```python
from build123d import *

# Parameters (mm, degrees)
F3_DEPTH = 67


with BuildPart() as f1:
    # F0 (on Right) → F1 (revolve)
    with BuildSketch(Plane.YZ):
        with BuildLine():
            ThreePointArc((-152.8260280422, -8.4497542544), (-145.7549602303, -5.5208220662), (-142.8260280422, 1.5502457456))
            ThreePointArc((-142.8260280422, 1.5502457456), (-145.7549602303, 8.6213135575), (-152.8260280422, 11.5502457456))
            Line((-152.8260280422, 11.5502457456), (-152.8260280422, -8.4497542544))
        make_face()
        with BuildLine():
            Line((-142.8260280422, -28.4497542544), (-142.8260280422, 1.5502457456))
            ThreePointArc((-142.8260280422, 1.5502457456), (-145.7549602303, -5.5208220662), (-152.8260280422, -8.4497542544))
            Line((-152.8260280422, -8.4497542544), (-152.8260280422, -18.4497542544))
            ThreePointArc((-152.8260280422, -18.4497542544), (-145.7549602303, -21.3786864425), (-142.8260280422, -28.4497542544))
        make_face()
        with BuildLine():
            ThreePointArc((-152.8260280422, -38.4497542544), (-145.7549602303, -35.5208220662), (-142.8260280422, -28.4497542544))
            ThreePointArc((-142.8260280422, -28.4497542544), (-145.7549602303, -21.3786864425), (-152.8260280422, -18.4497542544))
            Line((-152.8260280422, -18.4497542544), (-152.8260280422, -38.4497542544))
        make_face()
    revolve(axis=Axis((0, -152.8260280422, -13.4497542544), (0, 0, -1)))


with BuildPart() as f3:
    # F2 (on Front) → F3 (new body)
    with BuildSketch(Plane.XZ):
        Polygon((10.0054517388, -37.7888888825), (10.0054517388, -17.7050014576), (3.4798011376, -37.7888888825), align=None)
    extrude(amount=-F3_DEPTH)


with BuildPart() as f1_1:
    # F4: moved
    add(f1.part.moved(Location((0, 154, 0))))


with BuildPart() as f3_1:
    # F5: moved
    add(f3.part.moved(Location((0, -25, 0))))


with BuildPart() as f1_2:
    add(f1_1.part)

    # F6: cut F3
    add(f3_1.part, mode=Mode.SUBTRACT)


solid = f1_2.part
```
Geometry: final body of the model. Coordinates: model frame, mm. Coordinates: 2 decimals unless noted, no trailing zeros. Order: outer loops, then holes, each group sorted by start corner. A loop starts at its lowest first (then second) coordinate and runs counter-clockwise, first axis right, second up. Notation, with made-up numbers: (9.5, 33.5) - (13.5, 33.5) arc R17 ccw to (13.5, 58.5) - close; hole circle Ø8 at (-39.5, 27.25). An arc over 180 degrees is marked (long way). Return JSON: item names as keys, results as strings. Group by question number.
1. Cut plane D-D (x = 0). Output: boundary loops of the cut face in (y, z), plus the area to 3 significant figures.
2. Cut plane A-A (y = 4.75). Output: boundary loops of the cut face in (x, z), plus the area to 3 significant figures.
3. Material intervals for line 1 along Z through (x, y) = (-4.75, 3.5); line 2 along X through (y, z) = (7, -0.5); line 3 along Y through (x, z) = (-2.25, -9), sorted ascending. Write a range as [from, to].
4. Cut plane C-C (z = -31). Output: boundary loops of the cut face in (x, y).
5. Cut plane B-B (x = 5.25). Output: boundary loops of the cut face in (y, z) (3 decimals), plus the area to 3 significant figures.
6. Pin query (flat end, axial travel): pin 1 (1 mm diameter, centred on x = 2, y = 3, fed in from -Z); pin 2 (8 mm diameter, centred on y = 2.5, z = -7, fed in from +X); pin 3 (6 mm diameter, centred on x = 7, z = -32, fed in from -Y); pin 4 (3 mm diameter, centred on x = -2, y = 4.5, fed in from +Z). Return the tip coordinate at first contact, or that it passes through.
Resolved:
{
 "1": {"outline": "(-8.83, -28.45) arc R10 ccw to (11.17, -28.45) - (11.17, 1.55) arc R10 ccw to (-8.83, 1.55) - close", "area": "914 mm²"},
 "2": {"outline": "(-9.34, -28.45) arc R9.34 ccw to (3.73, -37.01) - (9.34, -19.76) - (9.34, 1.55) arc R9.34 ccw to (-9.34, 1.55) - close", "area": "799 mm²"},
 "3": {"line 1": "z = [-36.94, 10.04]", "line 2": "x = [-8.13, 8.13]", "line 3": "y = [-8.57, 10.92]"},
 "4": {"outline": "(5.69, -6.65) - (5.69, 9) arc R9.67 ccw (long way) to start"},
 "5": {"outline": "(-7.337, -28.45) arc R8.511 ccw to (-6.396, -32.341) - (8.743, -32.341) arc R8.511 ccw to (9.685, -28.45) - (9.685, 1.55) arc R8.511 ccw to (-7.337, 1.55) - close", "area": "688 mm²"},
 "6": {"pin 1": "stops at z = -38.2", "pin 2": "stops at x = 10", "pin 3": "stops at y = -7.57", "pin 4": "stops at z = 11.26"}
}
